from build123d import *

# Parameters (mm, degrees)
SKETCH2_W            = 540
SKETCH2_H            = 640
BOSS_EXTRUDE1_DEPTH  = 3.175
SKETCH3_W            = 45
SKETCH3_H            = 50
CUT_EXTRUDE1_DEPTH   = 838.382875765
FILLET1_R            = 10
FILLET2_R            = 3.175
M5_CLEARANCE_HOLE1_D = 5.8
LPATTERN1_COUNT      = 4
LPATTERN1_PITCH      = 125
M5_CLEARANCE_HOLE2_D = 5.8
LPATTERN2_COUNT      = 4
LPATTERN2_PITCH      = 125


with BuildPart() as part:
    # Sketch2 → Boss-Extrude1 (new body)
    with BuildSketch(Plane.XY):
        with Locations((270, 320)):
            Rectangle(SKETCH2_W, SKETCH2_H)
    extrude(amount=BOSS_EXTRUDE1_DEPTH)

    # Sketch3 → Cut-Extrude1 (cut, through all)
    with BuildSketch(Plane.XY.offset(3.175)):
        with Locations((22.5, 615)):
            Rectangle(SKETCH3_W, SKETCH3_H)
        Polygon((0, 121), (61, 121), (61, 90.5), (31, 60.5), (61, 30.5), (61, 0), (0, 0), align=None)
        Polygon((540, 0), (540, 121), (479, 121), (479, 90.5), (509, 60.5), (479, 30.5), (479, 0), align=None)
        with Locations((517.5, 615)):
            Rectangle(SKETCH3_W, SKETCH3_H)
    extrude(amount=-CUT_EXTRUDE1_DEPTH, mode=Mode.SUBTRACT)

    # Fillet1
    fillet1_edges = [part.edges().sort_by_distance(p)[0] for p in [
        (31, 60.5, 1.5875),
        (509, 60.5, 1.5875),
    ]]
    fillet(fillet1_edges, radius=FILLET1_R)

    # Fillet2
    fillet2_edges = [part.edges().sort_by_distance(p)[0] for p in [
        (45, 590, 1.5875),
        (61, 121, 1.5875),
        (479, 121, 1.5875),
        (495, 590, 1.5875),
    ]]
    fillet(fillet2_edges, radius=FILLET2_R)

    # M5 Clearance Hole1 (through all)
    with Locations(Plane(origin=(82.5, 10, 3.175), x_dir=(1, 0, 0), z_dir=(0, 0, 1))):
        with Locations((0, 0), (0, 100), (0, 620)):
            m5_clearance_hole1 = Hole(M5_CLEARANCE_HOLE1_D / 2)

    # LPattern1: M5 Clearance Hole1 ×4
    with Locations(*[(i * LPATTERN1_PITCH, 0, 0) for i in range(1, LPATTERN1_COUNT)]):
        add(m5_clearance_hole1, mode=Mode.SUBTRACT)

    # M5 Clearance Hole2 (through all)
    with Locations(Plane(origin=(10, 168, 3.175), x_dir=(1, 0, 0), z_dir=(0, 0, 1))):
        with Locations((0, 0), (520, 0)):
            m5_clearance_hole2 = Hole(M5_CLEARANCE_HOLE2_D / 2)

    # LPattern2: M5 Clearance Hole2 ×4
    with Locations(*[(0, i * LPATTERN2_PITCH, 0) for i in range(1, LPATTERN2_COUNT)]):
        add(m5_clearance_hole2, mode=Mode.SUBTRACT)


solid = part.part
Model file for the job. Use its own axes, mm. Give positions to 0.01 mm unless a question says otherwise; leave off trailing zeros. One line per item, written item: value.
Item 1: Pin check, flat tip, straight feed: pin 1 Ø1 at (x, z) = (26, 2) entering from +Y. Stop position of the tip, or through.
Response values:
pin 1: y = 590
Item 2: Two-plate mould, pull along Y, no slides. Class faces 1 (the flat face through (49.7, 79.2, 1.6)), 2 (the flat face through (266, 324, 3.175)), 3 (the flat face through (49.4, 42.1, 1.6)), 4 (the flat face through (490.3, 79.2, 1.6)): released by +Y, released by -Y, zero draft, split by the parting line, or undercut.
Response values:
face 1: undercut
face 2: zero draft
face 3: released by -Y
face 4: undercut
Item 3: Wall check: line 1 (Y direction, x = 530, z = 1); line 2 (Y direction, x = 332.5, z = 1.6); line 3 (X direction, y = 290.5, z = 1.1). Give the ranges that are in metal, low to high.
Response values:
line 1: 121 to 165.1, 170.9 to 290.1, 295.9 to 415.1, 420.9 to 540.1, 545.9 to 590
line 2: 0 to 7.1, 12.9 to 107.1, 112.9 to 627.1, 632.9 to 640
line 3: 0 to 8.53, 11.47 to 528.53, 531.47 to 540
Item 4: Slice it at A-A (z = 2.45). Give the number of separate pieces and of enclosed holes in the cut face, then the cut area to 3 significant figures.
Response values:
separate pieces: 1
enclosed holes: 20
area: 328,000 mm2
